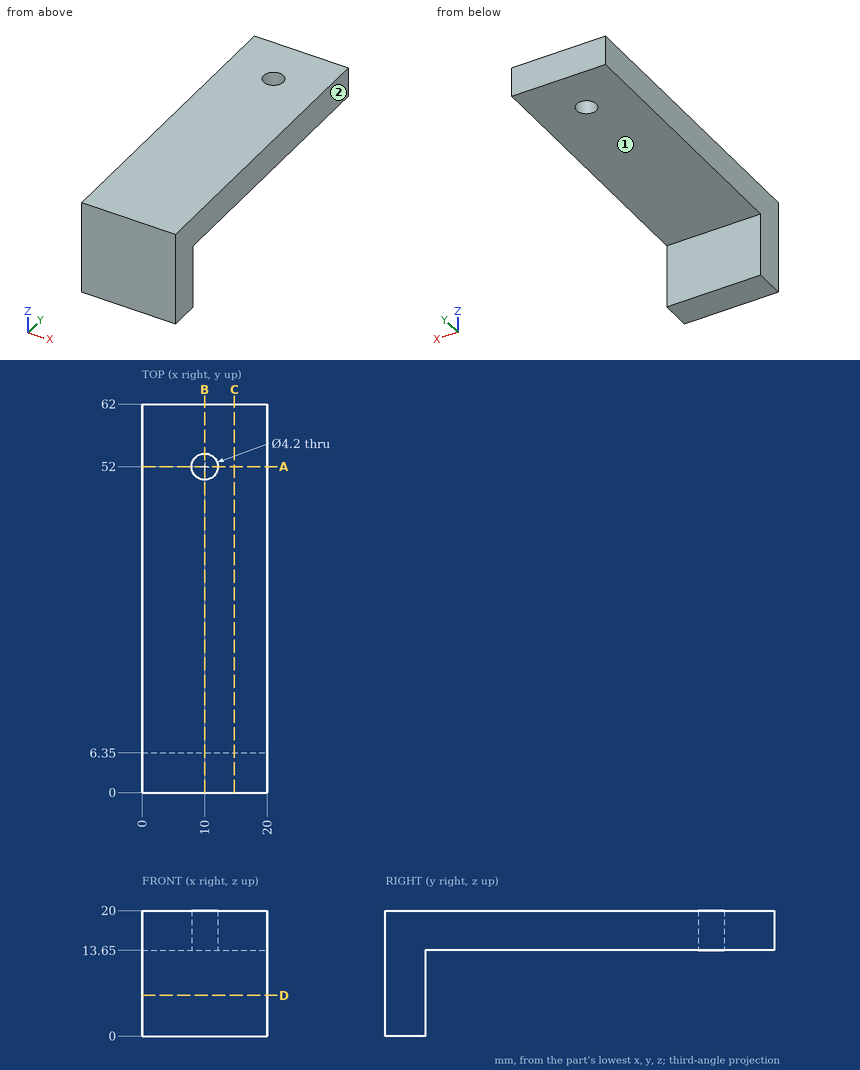
Input: dimensioned drawing with shaded views. Units: mm. Origin: part minimum x, y, z. A direction names the side the tool comes from. Give positions to 0.01 mm unless a question says otherwise; leave off trailing zeros. Loops run counter-clockwise (first coordinate to the right, second up) from the corner with the lowest first, then second, coordinate; pieces in that order, holes last. Notation, with made-up numbers: M 54,-34.75 L 73,-34.75 A8 cw 73,-30.75 Z; hole C 84.25,-23.75 d8. An arc over 180 degrees is marked long. Put each result on its own line as item: value.
1) Material intervals for L1, parallel to Y at x = 10, z = 17.5; L2, parallel to Y at x = 7.25, z = 1.5; L3, parallel to Z at x = 15, y = 31, sorted ascending. Write a range as from..to.
Computed values:
L1: y = 0..49.9, 54.1..62
L2: y = 0..6.35
L3: z = 13.65..20
2) Cut plane D-D, the plane z = 6.5. Return the cut outline in (x, y).
Computed values:
outline: M 0,0 L 20,0 L 20,6.35 L 0,6.35 Z
3) First-contact query: P1, Ø6.5, axis at x = 10, y = 52, coming from the -Z side; P2, Ø10, axis at y = 35, z = 5.5, coming from the -X side. Flat tips, straight axial feed; report the tip coordinate or a pass-through.
Computed values:
P1: stops at z = 13.65
P2: passes through
4) Cut plane C-C, the plane x = 14.75. Return the cut outline in (y, z), plus the area to 3 significant figures.
Computed values:
outline: M 0,0 L 6.35,0 L 6.35,13.65 L 62,13.65 L 62,20 L 0,20 Z
area: 480 mm^2
5) Cut plane A-A, the plane y = 52. Return the cut outline in (x, z).
Computed values:
outline: M 0,13.65 L 7.9,13.65 L 7.9,20 L 0,20 Z; M 12.1,13.65 L 20,13.65 L 20,20 L 12.1,20 Z
6) Cut plane B-B, the plane x = 10. Return the cut outline in (y, z).
Computed values:
outline: M 0,0 L 6.35,0 L 6.35,13.65 L 49.9,13.65 L 49.9,20 L 0,20 Z; M 54.1,13.65 L 62,13.65 L 62,20 L 54.1,20 Z
7) Reachability of the marked faces 1 and 2 from +Z, -Z, +X, -X, +Y, -Y: full face, straight path, thin tool, end or side. Return the list, or none.
Computed values:
face 1: -Z, +X, -X, +Y
face 2: +Z, -Z, +X, +Y, -Y
